```python
from build123d import *

# Parameters (mm, degrees)
SKETCH1_R           = 2.1
BOSS_EXTRUDE1_DEPTH = 11.38
FILLET1_R           = 4


with BuildPart() as part:
    # Sketch1 → Boss-Extrude1 (new body)
    with BuildSketch(Plane(origin=(0, 0, 0), x_dir=(1, 0, 0), z_dir=(0, 1, 0))):
        Polygon((0, 0), (64, 0), (64, 67.63), (28.533540344, 67.63), align=None)
        with Locations(Location((16, 8, 0), (0, 0, 270))):
            Circle(SKETCH1_R, mode=Mode.SUBTRACT)
        with Locations(Location((48, 8, 0), (0, 0, 270))):
            Circle(SKETCH1_R, mode=Mode.SUBTRACT)
        with Locations(Location((36.475395885, 51.63, 0), (0, 0, 270))):
            Circle(SKETCH1_R, mode=Mode.SUBTRACT)
    extrude(amount=BOSS_EXTRUDE1_DEPTH)

    # Fillet1
    fillet1_edges = [part.edges().sort_by_distance(p)[0] for p in [
        (28.533540344, 5.69, -67.63),
        (64, 5.69, -67.63),
    ]]
    fillet(fillet1_edges, radius=FILLET1_R)


solid = part.part
```
The model under review builds one solid part; all positions refer to its coordinate system, in mm. Give positions to 0.01 mm unless a question says otherwise; leave off trailing zeros. Write each loop counter-clockwise with the first axis right and the second up, starting at its lowest first coordinate (ties: lowest second). Pieces come first, ordered by that corner, then holes. Notation, with made-up numbers: M 13,28 L 72,28 A13 cw 72,48 Z; hole C -15,72.5 d3. An arc over 180 degrees is marked long. Write each question's results on one line, items separated by ' | '. Start each with the question number.
1. We need section D-D (z = -51.63). Write out the cut boundary in (x, y).
2. Insertion check: pin 1 Ø10 at (x, z) = (13, -15.5) entering from -Y. The pin has a flat end and moves straight along its axis. Give the tip position at first contact, or say it passes through.
3. We need section A-A (x = 48). Write out the cut boundary in (y, z).
4. We need section C-C (y = 5.5). Write out the cut boundary in (x, z).
5. Mouldability with a two-part tool opening along X and no side actions: class faces 1 (the flat face through (64, 6, -31)), 2 (the cylindrical face through (28.949, 5.77, -66.945)), 3 (the cylindrical face through (17.419, 5.61, -9.548)) as released by +X, released by -X, zero draft, split by the parting line, or undercut.
6. We need section B-B (z = -8). Write out the cut boundary in (x, y), and give its area (3 significant figures).
7. For probe 1 along X at (y, z) = (6.25, -8); probe 2 along X at (y, z) = (7.5, -27); probe 3 along Z at (x, y) = (48.5, 7.5), list the stretches that pass through material, from the lowest coordinate up. Write a range as [from, to].
Results found:
1) outline: M 21.78,0 L 34.38,0 L 34.38,11.38 L 21.78,11.38 Z; M 38.58,0 L 64,0 L 64,11.38 L 38.58,11.38 Z
2) pin 1: stops at y = 0
3) outline: M 0,-67.63 L 11.38,-67.63 L 11.38,-10.1 L 0,-10.1 Z; M 0,-5.9 L 11.38,-5.9 L 11.38,0 L 0,0 Z
4) outline: M 0,0 L 27.5,-65.18 A4 ccw 31.19,-67.63 L 60,-67.63 A4 ccw 64,-63.63 L 64,0 Z; hole C 16,-8 d4.2; hole C 36.48,-51.63 d4.2; hole C 48,-8 d4.2
5) face 1: released by +X | face 2: released by -X | face 3: undercut
6) outline: M 3.38,0 L 13.9,0 L 13.9,11.38 L 3.38,11.38 Z; M 18.1,0 L 45.9,0 L 45.9,11.38 L 18.1,11.38 Z; M 50.1,0 L 64,0 L 64,11.38 L 50.1,11.38 Z | area: 594 mm^2
7) probe 1: x = [3.38, 13.9], [18.1, 45.9], [50.1, 64] | probe 2: x = [11.39, 64] | probe 3: z = [-67.63, -10.04], [-5.96, 0]
